```python
from build123d import *

# Parameters (mm, degrees)
SKETCH1_R                = 10
BOSS_EXTRUDE1_DEPTH      = 20
BOSS_EXTRUDE2_DEPTH      = 20
BOSS_EXTRUDE3_DEPTH      = 10
BOSS_EXTRUDE3_DEPTH_BACK = 15
CUT_EXTRUDE1_DEPTH       = 20
CIRPATTERN1_COUNT        = 18
SKETCH11_R               = 10
CUT_EXTRUDE3_DEPTH       = 33
SKETCH12_R               = 10
CUT_EXTRUDE4_DEPTH       = 5


with BuildPart() as part:
    # Sketch1 → Boss-Extrude1 (new body)
    with BuildSketch(Plane.XY):
        with BuildLine():
            Line((-71.370560529, 20), (276.629439471, 20))
            ThreePointArc((276.629439471, 20), (296.629439471, 0), (276.629439471, -20))
            Line((276.629439471, -20), (-71.370560529, -20))
            ThreePointArc((-71.370560529, -20), (-91.370560529, 0), (-71.370560529, 20))
        make_face()
        with Locations((-71.370560529, 0)):
            Circle(SKETCH1_R, mode=Mode.SUBTRACT)
        with Locations((276.629439471, 0)):
            Circle(SKETCH1_R, mode=Mode.SUBTRACT)
    extrude(amount=BOSS_EXTRUDE1_DEPTH)

    # Sketch2 → Boss-Extrude2 (add)
    with BuildSketch(Plane(origin=(0, 0, 0), x_dir=(-1, 0, 0), z_dir=(0, 0, -1))):
        with BuildLine():
            Line((71.370560529, -20), (71.370560529, -25))
            ThreePointArc((71.370560529, -25), (64.900084402, -24.148145657), (58.870560529, -21.650635095))
            Line((58.870560529, -21.650635095), (62.564306071, -17.956889553))
            ThreePointArc((62.564306071, -17.956889553), (66.850482602, -19.482527955), (71.370560529, -20))
        make_face()
    extrude(amount=BOSS_EXTRUDE2_DEPTH)

    # Sketch6 → Boss-Extrude3 (add, two sides)
    with BuildSketch(Plane.XY.offset(15)) as boss_extrude3_sk:
        Polygon((-65.848114546, 25.970849484), (-62.185743951, 14.6961629), (-57.298605127, 22.515827849), (-57.713272426, 10.668483548), (-50.44638121, 16.345065077), (-54.888071406, 5.354027631), (-46.117922126, 8.20284623), (-54.050901831, -0.606203036), (-44.835303924, -0.928756935), (-55.302738705, -6.49331667), (-46.753229286, -9.948338305), (-58.492592027, -11.597240483), (-51.64036811, -17.768003255), (-63.235718409, -15.302365936), (-58.907259326, -23.444584784), (-68.960026809, -17.161800219), (-67.677408606, -26.293403383), (-74.97508115, -16.951268114), (-76.893006513, -25.970849484), (-80.555377108, -14.6961629), (-85.442515932, -22.515827849), (-85.027848633, -10.668483548), (-92.294739849, -16.345065077), (-87.853049653, -5.354027631), (-96.623198932, -8.20284623), (-88.690219228, 0.606203036), (-97.905817135, 0.928756935), (-87.438382354, 6.49331667), (-95.987891773, 9.948338305), (-84.248529032, 11.597240483), (-91.100752949, 17.768003255), (-79.50540265, 15.302365936), (-83.833861733, 23.444584784), (-73.78109425, 17.161800219), (-75.063712453, 26.293403383), (-67.766039909, 16.951268114), align=None)
    extrude(amount=BOSS_EXTRUDE3_DEPTH)
    extrude(boss_extrude3_sk.sketch, amount=-BOSS_EXTRUDE3_DEPTH_BACK)

    # Sketch10 → Cut-Extrude1 (cut)
    with BuildSketch(Plane.XY.offset(20)):
        with BuildLine():
            Line((-77.019410052, 19.185684743), (-73.78109425, 17.161800219))
            Line((-73.78109425, 17.161800219), (-74.152438156, 19.805583982))
            ThreePointArc((-74.152438156, 19.805583982), (-75.597303819, 19.548264403), (-77.019410052, 19.185684743))
        make_face()
    cut_extrude1 = extrude(amount=-CUT_EXTRUDE1_DEPTH, mode=Mode.SUBTRACT)

    # CirPattern1: Cut-Extrude1 ×18 about axis, 9 skipped
    cirpattern1_axis = Axis((-71.370560529, 0, 20), (0, 0, -1))
    add([cut_extrude1.rotate(cirpattern1_axis, i * 360 / CIRPATTERN1_COUNT) for i in range(1, CIRPATTERN1_COUNT) if i not in (1, 2, 3, 4, 5, 6, 7, 8, 9)], mode=Mode.SUBTRACT)

    # Sketch11 → Cut-Extrude3 (cut)
    with BuildSketch(Plane.XY.offset(25)):
        with Locations((-71.370560529, 0)):
            Circle(SKETCH11_R)
    extrude(amount=-CUT_EXTRUDE3_DEPTH, mode=Mode.SUBTRACT)

    # Sketch12 → Cut-Extrude4 (cut)
    with BuildSketch(Plane.XY.offset(25)):
        Polygon((-97.905817135, 0.928756935), (-88.690219228, 0.606203036), (-96.623198932, -8.20284623), (-87.853049653, -5.354027631), (-92.294739849, -16.345065077), (-85.027848633, -10.668483548), (-85.442515932, -22.515827849), (-80.555377108, -14.6961629), (-76.893006513, -25.970849484), (-74.97508115, -16.951268114), (-67.677408606, -26.293403383), (-68.960026809, -17.161800219), (-58.907259326, -23.444584784), (-63.235718409, -15.302365936), (-51.64036811, -17.768003255), (-58.492592027, -11.597240483), (-46.753229286, -9.948338305), (-55.302738705, -6.49331667), (-44.835303924, -0.928756935), (-54.050901831, -0.606203036), (-46.117922126, 8.20284623), (-54.888071406, 5.354027631), (-50.44638121, 16.345065077), (-57.713272426, 10.668483548), (-57.298605127, 22.515827849), (-62.185743951, 14.6961629), (-65.848114546, 25.970849484), (-67.766039909, 16.951268114), (-75.063712453, 26.293403383), (-73.78109425, 17.161800219), (-83.833861733, 23.444584784), (-79.50540265, 15.302365936), (-91.100752949, 17.768003255), (-84.248529032, 11.597240483), (-95.987891773, 9.948338305), (-87.438382354, 6.49331667), align=None)
        with Locations((-71.370560529, 0)):
            Circle(SKETCH12_R, mode=Mode.SUBTRACT)
    extrude(amount=-CUT_EXTRUDE4_DEPTH, mode=Mode.SUBTRACT)


solid = part.part
```
Can you work these out from the model? Positions are in its coordinate system, mm. A direction names the side the tool comes from. Coordinates: 2 decimals unless noted, no trailing zeros. Loops run counter-clockwise (first coordinate to the right, second up) from the corner with the lowest first, then second, coordinate; pieces in that order, holes last. Notation, with made-up numbers: (49.5, -28) -> (64.5, -28) arc R25 ccw to (64.5, -12) -> close; hole circle Ø7 at (84.25, 35.5). An arc over 180 degrees is marked (long way). Put each result on its own line as item: value. Start each with the question number.
Q1. I want a section at B-B (x = 100). Write out the boundary of the cut face in (y, z).
Q2. I'm going to push flat-ended pins straight in: P1, Ø1.5, axis at x = -61, z = 11.5, coming from the +Y side; P2, Ø1.5, axis at y = -4.5, z = 6, coming from the -X side; P3, Ø3, axis at x = 226.5, y = -14.5, coming from the -Z side. Where does each tip first touch, or does it pass through?
Q3. For faces 4 (the face through (-66.79, -19.47, -9.86)), 5 (the face through (-61.83, 3, 10.14)), 6 (the face through (-68.126, -23.103, 9.86)), which set-ups out of +Z, -Z, +X, -X, +Y, -Y let a thin tool reach every point of the face, with its end or its side?
Q4. If I drill on line 1 (X direction, y = -1.5, z = 8); line 2 (X direction, y = -22, z = 11.5); line 3 (Z direction, x = 205.5, y = 12), over which ranges is the centre line in solid material (lowest first)? Write a range as [from, to].
Q5. Thinking about a two-plate mould opening in X: for faces 1 (the face through (-64.99, -24.17, -9.86)), 2 (the face through (107, 20, 10)), 3 (the face through (-72.64, 23.19, 9.86)), which applies, pulls with the +X half, pulls with the -X half, needs draft (parallel to the pull), parting line crosses it, or undercut?
Q6. I want a section at C-C (z = -15). Write out the boundary of the cut face in (x, y), plus the area to 3 significant figures.
Q7. I want a section at A-A (z = 7). Count the separate pieces of the cut face and the enclosed holes in it, plus the area to 3 significant figures.
Taken from the geometry:
1. outline: (-20, 0) -> (20, 0) -> (20, 20) -> (-20, 20) -> close
2. P1: stops at y = 20
2. P2: stops at x = -93.96
2. P3: stops at z = 0
3. face 4: -Z, -X, +Y
3. face 5: +Z, -Z
3. face 6: +Z
4. line 1: x = [-90.59, -81.26], [-61.48, 266.74], [286.52, 296.57]
4. line 2: x = [-85.42, -85.12], [-78.18, -76.05], [-71.03, -68.28], [-61.22, -59.68]
4. line 3: z = [0, 20]
5. face 1: pulls with the +X half
5. face 2: needs draft
5. face 3: undercut
6. outline: (-71.37, -25) arc R25 ccw to (-58.87, -21.65) -> (-62.56, -17.96) arc R20 cw to (-71.37, -20) -> close
6. area: 55.5 mm2
7. separate pieces: 1
7. enclosed holes: 2
7. area: 14,700 mm2
